```python
from build123d import *

# Parameters (mm, degrees)
BOSS_EXTRUDE1_DEPTH = 25.4
SKETCH2_R           = 11.1252
BOSS_EXTRUDE2_DEPTH = 88.9
SKETCH3_R           = 3.175
CUT_EXTRUDE1_DEPTH  = 28.972160483


with BuildPart() as part:
    # Sketch1 → Boss-Extrude1 (new body)
    with BuildSketch(Plane.XY):
        Polygon((0, 0), (5.588, 0), (5.588, 3.556), (-46.6344, 3.556), (-46.6344, -120.904), (-51.7144, -120.904), (-51.7144, 6.096), (8.128, 6.096), (8.128, -2.54), (0, -2.54), align=None)
    extrude(amount=BOSS_EXTRUDE1_DEPTH)

    # Sketch2 → Boss-Extrude2 (add)
    with BuildSketch(Plane.ZY.offset(51.7144)):
        with Locations((12.7, -109.7788)):
            Circle(SKETCH2_R)
    extrude(amount=BOSS_EXTRUDE2_DEPTH)

    # Sketch3 → Cut-Extrude1 (cut, through all)
    with BuildSketch(Plane(origin=(0, -40.672695638, -40.672695638), x_dir=(1, 0, 0), z_dir=(0, 0.707106781, 0.707106781))):
        with Locations((-134.2644, -86.605590032)):
            Circle(SKETCH3_R)
    extrude(amount=-CUT_EXTRUDE1_DEPTH, mode=Mode.SUBTRACT)


solid = part.part
```
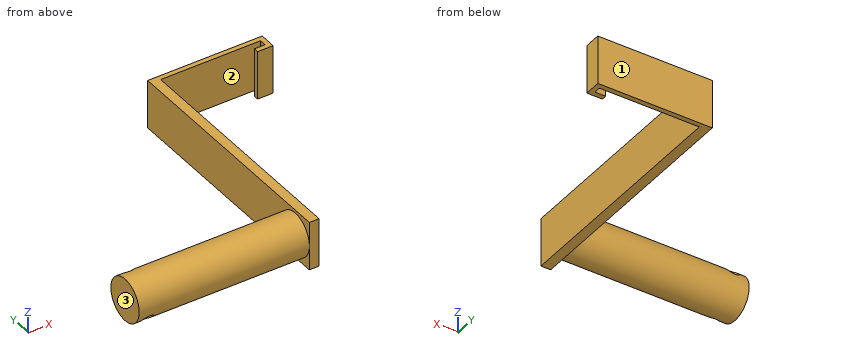
Geometry check sheet. Reference: the model listing, model coordinates, mm. Face numbers are marked on the shaded views. Round coordinates to 2 decimals unless told otherwise and drop trailing zeros. Order: outer loops, then holes, each group sorted by start corner. A loop starts at its lowest first (then second) coordinate and runs counter-clockwise, first axis right, second up. Notation, with made-up numbers: (-1, 70.5) - (4, 70.5) arc R18 cw to (4, 92.5) - close; hole circle Ø3 at (-12.75, 26.25). An arc over 180 degrees is marked (long way). Use a Markdown table: item, result. Add a question column.
1) Thickness scan on line 1 along X through (y, z) = (-1, 2); line 2 along X through (y, z) = (-71, 17); line 3 along Z through (x, y) = (-128.5, -115). Record the ranges inside material, lowest first.
2) Section check C-C (x = -56). Record the cut outline in (y, z), then the cut area to 3 significant figures.
3) Section check A-A (x = -27). Record the cut outline in (y, z).
4) Gauge pin test, flat ends, axial feed: P1, Ø1.3, axis at y = -1, z = 6.5, coming from the -X side; P2, Ø6.5, axis at x = 3.5, z = 16.5, coming from the -Y side; P3, Ø2, axis at x = -111, z = 16.5, coming from the +Y side. Record the tip position at first contact, or that the pin passes through.
5) Mould release check, pull along X, two halves, no side actions. Record for the marked faces 1, 2 and 3: released by +X, released by -X, zero draft, split by the parting line, or undercut.
6) Section check B-B (y = -86.5). Record the cut outline in (x, z).
Established:
| question | item | result |
|---|---|---|
| 1 | line 1 | -51.71 to -46.63, 0 to 8.13 |
| 1 | line 2 | -51.71 to -46.63 |
| 1 | line 3 | 2.88 to 22.52 |
| 2 | outline | circle Ø22.25 at (-109.78, 12.7) |
| 2 | area | 389 mm2 |
| 3 | outline | (3.56, 0) - (6.1, 0) - (6.1, 25.4) - (3.56, 25.4) - close |
| 4 | P1 | x = -51.71 |
| 4 | P2 | y = -2.54 |
| 4 | P3 | y = -99.01 |
| 5 | face 1 | zero draft |
| 5 | face 2 | undercut |
| 5 | face 3 | released by -X |
| 6 | outline | (-51.71, 0) - (-46.63, 0) - (-46.63, 25.4) - (-51.71, 25.4) - close |
